```python
from build123d import *


with BuildPart() as part:
    # По траектории1: sweep along a path in Эскиз1
    with BuildLine(Plane.XY) as sweep_1_path:
        Line((-161.247058824, 47.195190653), (3.1, 16.714963356))
        ThreePointArc((3.1, 16.714963356), (17, 0), (3.1, -16.714963356))
        Line((3.1, -16.714963356), (-161.247058824, -47.195190653))
        ThreePointArc((-161.247058824, -47.195190653), (-218, 0), (-161.247058824, 47.195190653))
    # Эскиз2 → По траектории1 (sweep)
    with BuildSketch(Plane(origin=(0, 0, 0), x_dir=(1, 0, 0), z_dir=(0, 1, 0))):
        Polygon((-212.5, 3.05389582), (-216, 1.78), (-212.5, 0.50610418), (-212.5, -0.50610418), (-216, -1.78), (-212.5, -3.05389582), (-212.5, -4.06610418), (-216, -5.34), (-212.5, -6.61389582), (-212.5, -7.62610418), (-216, -8.9), (-216, -9.4), (-218, -9.4), (-218, 9.4), (-216, 9.4), (-216, 8.9), (-212.5, 7.62610418), (-212.5, 6.61389582), (-216, 5.34), (-212.5, 4.06610418), align=None)
    sweep(path=sweep_1_path.line)


solid = part.part
```
The model under review builds one solid part; all positions refer to its coordinate system, in mm. A direction names the side the tool comes from. Round coordinates to 2 decimals unless told otherwise and drop trailing zeros. Use one line per item in the form item = value.
Q1. Insertion check: pin 1 Ø3 at (x, z) = (-153, -1.5) entering from -Y; pin 2 Ø1 at (x, z) = (-13, 3) entering from -Y; pin 3 Ø12 at (x, y) = (-115.5, 29) entering from +Z. Each pin has a flat end and moves straight along its axis. Give the tip position at first contact, or say it passes through.
Answer key:
pin_1 = -45.94
pin_2 = -19.79
pin_3 = 8.34
Q2. Tool access review of faces 3 (the flat face through (-78.611, 28.031, -4.694)), 4 (the flat face through (-80.589, -30.202, 9.154)), 5 (the flat face through (-78.926, 26.334, -3.553)): name each direction out of +Z, -Z, +X, -X, +Y, -Y from which nothing blocks a thin tool from reaching the whole face with its end or side.
Answer key:
face_3 = none
face_4 = +Z
face_5 = +Z, -Z
Q3. Draft analysis for pull direction X (two halves, no side actions). For faces 1 (the flat face through (-80.903, -28.505, 4.712)), 2 (the flat face through (-78.602, 28.079, 4.712)), state which applies: +X half, -X half, draft (parallel to the pull), parting line (faces both ways), or undercut.
Answer key:
face_1 = undercut
face_2 = undercut
Q4. For line 1 (Y direction, x = -170, z = -3.55); line 2 (X direction, y = 0, z = -7.3); line 3 (Y direction, x = -170, z = 9.35), list the stretches that pass through material, from the lowest coordinate up. Write a range as [from, to].
Answer key:
line_1 = [-48, -42.5], [42.5, 48]
line_2 = [-218, -212.5], [11.5, 17]
line_3 = [-48, -46], [46, 48]
